Study the drawing (mm; zero at the part's minimum x, y, z) and answer. Round coordinates to 2 decimals unless told otherwise and drop trailing zeros. Write each loop counter-clockwise with the first axis right and the second up, starting at its lowest first coordinate (ties: lowest second). Pieces come first, ordered by that corner, then holes.
(1) The mould has two halves that part along X. Classify the marked faces 1 and 2: +X half, -X half, draft (parallel to the pull), parting line (faces both ways), or undercut.
(2) A cutting plane is placed at C-C, the plane z = 362. Give the number of separate pieces and of enclosed holes in the cut face.
(3) A cutting plane is placed at A-A, the plane y = 132.5. Give the vertices of the cut face in (x, z), and give its area (3 significant figures).
(4) Find the intervals of material crossed by probe 1 along Y at (x, z) = (219, 301.5); probe 2 along X at (y, z) = (251.5, 116.5) (1 decimal); probe 3 along Z at (x, y) = (169, 188), in increasing order.
(5) A cutting plane is placed at B-B, the plane x = 214.5. Give the vertices of the cut face in (y, z), and give its area (3 significant figures).
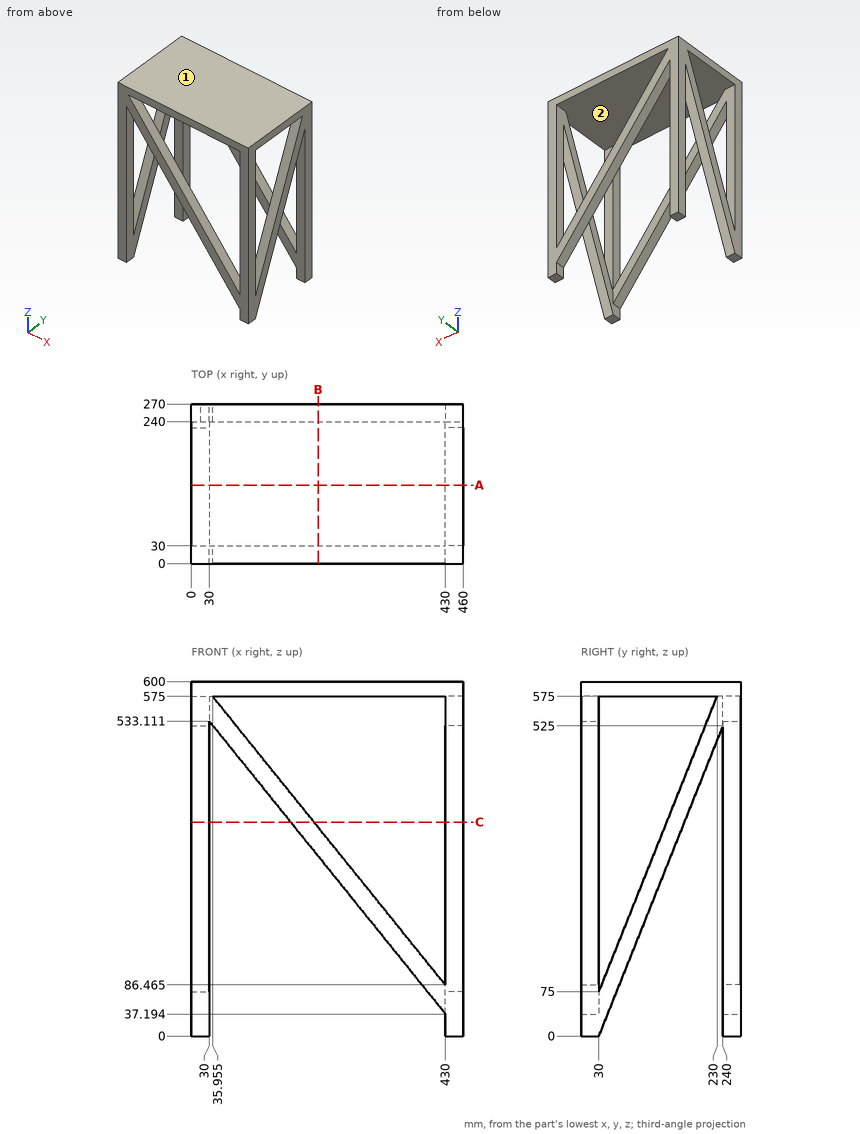
Solutions:
1. face 1: draft
1. face 2: undercut
2. separate pieces: 8
2. enclosed holes: 0
3. outline: (0, 256.25) - (30, 256.25) - (30, 331.25) - (0, 331.25) - close; (0, 575) - (460, 575) - (460, 600) - (0, 600) - close; (430, 256.25) - (460, 256.25) - (460, 331.25) - (430, 331.25) - close
3. area: 16,000 mm2
4. probe 1: y = 0 to 30, 240 to 270
4. probe 2: x = 0 to 30, 366 to 405.8, 430 to 460
4. probe 3: z = 575 to 600
5. outline: (0, 304.37) - (30, 304.37) - (30, 353.64) - (0, 353.64) - close; (0, 575) - (270, 575) - (270, 600) - (0, 600) - close; (240, 304.37) - (270, 304.37) - (270, 353.64) - (240, 353.64) - close
5. area: 9,710 mm2
